from build123d import *

# Parameters (mm, degrees)
F0_R     = 19.05
F1_DEPTH = 57.15
F2_R     = 7.9375
F3_DEPTH = 44.45
F4_R     = 2.54
F5_SIZE  = 0.3


with BuildPart() as f1:
    # F0 (on Top) → F1 (new body)
    with BuildSketch(Plane.XY):
        Circle(F0_R)
    extrude(amount=F1_DEPTH)

    # F2 (on face) → F3 (cut)
    with BuildSketch(Plane.XY.offset(57.15)):
        Circle(F2_R)
    extrude(amount=-F3_DEPTH, mode=Mode.SUBTRACT)

    # F4
    f4_edges = [f1.edges().sort_by_distance(p)[0] for p in [
        (-19.05, 0, 0),
        (-19.05, 0, 57.15),
    ]]
    fillet(f4_edges, radius=F4_R)

    # F5
    f5_edges = [f1.edges().sort_by_distance(p)[0] for p in [
        (-7.9375, 0, 57.15),
        (-7.9375, 0, 12.7),
    ]]
    chamfer(f5_edges, length=F5_SIZE)


solid = f1.part
Geometry check sheet. Reference: the model listing, model coordinates, mm. A direction names the side the tool comes from. Give positions to 0.01 mm unless a question says otherwise; leave off trailing zeros. Loops run counter-clockwise (first coordinate to the right, second up) from the corner with the lowest first, then second, coordinate; pieces in that order, holes last. Notation, with made-up numbers: M 25,89.5 L 31,89.5 A25 ccw 31,113.5 Z; hole C 61,32 d10. An arc over 180 degrees is marked long. Write each question's results on one line, items separated by ' | '.
1) Thickness scan on line 1 (Y direction, x = 0, z = 38); line 2 (Z direction, x = -2.5, y = 2.5); line 3 (X direction, y = -3, z = 54.5). Record the ranges inside material, lowest first.
Answers follow:
line 1: -19.05 to -7.94, 7.94 to 19.05 | line 2: 0 to 12.7 | line 3: -18.81 to -7.35, 7.35 to 18.81
2) Release check for a two-part mould opening along Y. For faces 1 (the face through (0, 0, 12.7)), 2 (the face through (-15.12, -11.59, 28.21)), 3 (the face through (0, 0, 0)) record: +Y half, -Y half, draft (parallel to the pull), parting line (faces both ways), or undercut.
Answers follow:
face 1: undercut | face 2: parting line | face 3: draft
3) Section check A-A, the plane y = 0. Record the boundary of the cut face in (x, z).
Answers follow:
outline: M -19.05,2.54 A2.54 ccw -16.51,0 L 16.51,0 A2.54 ccw 19.05,2.54 L 19.05,54.61 A2.54 ccw 16.51,57.15 L 8.24,57.15 L 7.94,56.85 L 7.94,13 L 7.64,12.7 L -7.64,12.7 L -7.94,13 L -7.94,56.85 L -8.24,57.15 L -16.51,57.15 A2.54 ccw -19.05,54.61 Z
4) Tool access check on faces 4 (the face through (-1.72, -7.75, 35.23)), 5 (the face through (-8, -3, 57.15)). Record the directions out of +Z, -Z, +X, -X, +Y, -Y that give a thin tool (end or side, any length) a straight path to the whole face; none if there is none.
Answers follow:
face 4: +Z | face 5: +Z, +X, -X, +Y, -Y
5) Gauge pin test, flat ends, axial feed: pin 1 (2 mm diameter, centred on x = -4.5, z = 26.5, fed in from -Y); pin 2 (12 mm diameter, centred on y = 9, z = 45.5, fed in from +X); pin 3 (9.5 mm diameter, centred on x = 0, y = 0, fed in from +Z). Record the tip position at first contact, or that the pin passes through.
Answers follow:
pin 1: y = -18.73 | pin 2: x = 18.81 | pin 3: z = 12.7
6) Section check D-D, the plane z = 4. Record the boundary of the cut face in (x, y).
Answers follow:
outline: C 0,0 d38.1
